Geometry: final body of the model. Coordinates: model frame, mm. Face numbers are marked on the shaded views. Round coordinates to 2 decimals unless told otherwise and drop trailing zeros. Write each loop counter-clockwise with the first axis right and the second up, starting at its lowest first coordinate (ties: lowest second). Pieces come first, ordered by that corner, then holes. Notation, with made-up numbers: (-35.5, 49.25) -> (-3.5, 49.25) arc R24 ccw to (-3.5, 87.25) -> close; hole circle Ø3 at (-29.5, -37). An arc over 180 degrees is marked (long way). Use one line per item in the form item = value. Start each with the question number.
1. Cut plane A-A, the plane z = 210. Return the cut outline in (x, y).
2. Line query: L1, parallel to X at y = 183.5, z = 282; L2, parallel to Z at x = -108, y = 96.5; L3, parallel to Y at x = -107, z = 619.5. Output: solid intervals per line, ascending.
3. Cut plane B-B, the plane x = 62. Return the cut outline in (y, z), plus the area to 3 significant figures.
4. Cut plane C-C, the plane z = 409.5. Return the cut outline in (x, y), plus the area to 3 significant figures.
5. Draft query along Y for the marked faces 1, 2 and 3. Return one class per face: pulls with the +Y half, pulls with the -Y half, needs draft (parallel to the pull), parting line crosses it, or undercut.
6. Pin query (flat end, axial travel): pin 1 Ø10 at (x, z) = (94, 382) entering from +Y; pin 2 Ø1.5 at (x, z) = (-61.5, 582) entering from +Y; pin 3 Ø4 at (x, y) = (-74.5, 30.5) entering from -Z. Return the tip coordinate at first contact, or that it passes through.
7. Cut plane D-D, the plane y = 159. Return the cut outline in (x, z), plus the area to 3 significant figures.
```python
from build123d import *

# Parameters (mm, degrees)
F0_W      = 400
F0_H      = 400
F1_DEPTH  = 400
F2_W      = 300
F2_H      = 350
F3_DEPTH  = 400.001
F4_W      = 300
F4_H      = 350
F5_DEPTH  = 400.001
F8_W      = 400
F8_H      = 330.777927181
F9_DEPTH  = 50
F10_DEPTH = 9.0852224141
F11_W     = 300
F11_H     = 150
F12_DEPTH = 176.0726081542


with BuildPart() as f1:
    # F0 (on Top) → F1 (new body)
    with BuildSketch(Plane.XY):
        Rectangle(F0_W, F0_H)
    extrude(amount=F1_DEPTH)

    # F2 (on face) → F3 (cut, through all)
    with BuildSketch(Plane.XZ.offset(200)):
        with Locations((0, 175)):
            Rectangle(F2_W, F2_H)
    extrude(amount=-F3_DEPTH, mode=Mode.SUBTRACT)

    # F4 (on face) → F5 (cut, through all)
    with BuildSketch(Plane.YZ.offset(200)):
        with Locations((0, 175)):
            Rectangle(F4_W, F4_H)
    extrude(amount=-F5_DEPTH, mode=Mode.SUBTRACT)



with BuildPart() as f9:
    # F8 (on face) → F9 (new body)
    with BuildSketch(Plane(origin=(0, 125.5652334135, -22.1405384897), x_dir=(1, 0, 0), z_dir=(0, -0.984807753, 0.1736481777))):
        with Locations((0, 594.3105737075)):
            Rectangle(F8_W, F8_H)
    extrude(amount=F9_DEPTH)


with BuildPart() as f1_1:
    add(f1.part)
    # F10 (add, through all): a face of the model
    f10_faces = [f9.part.faces().sort_by_distance(p)[0] for p in [
        (0, 175.4264955469, 404.6059930296),
    ]]

    add(f9.part)  # F10 merges F9
    extrude(f10_faces, amount=F10_DEPTH)

    # F11 (on face) → F12 (cut, through all)
    with BuildSketch(Plane(origin=(0, 76.3248457628, -13.4581296064), x_dir=(1, 0, 0), z_dir=(0, -0.984807753, 0.1736481777))):
        with Locations((0, 494.8363877028)):
            Rectangle(F11_W, F11_H)
    extrude(amount=-F12_DEPTH, mode=Mode.SUBTRACT)


solid = f1_1.part
```
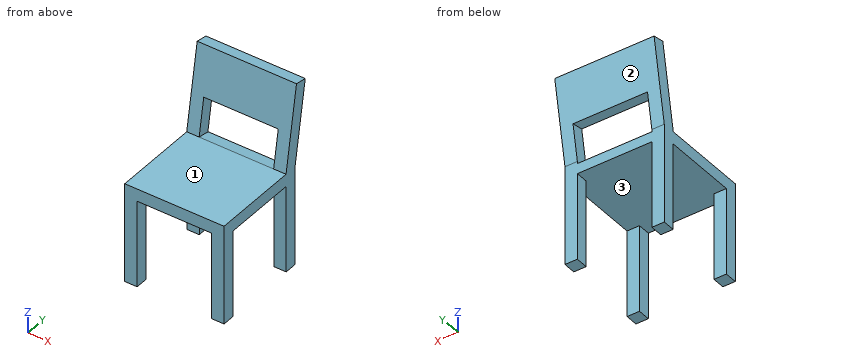
Outcome:
q1.outline = (-200, -200) -> (-150, -200) -> (-150, -150) -> (-200, -150) -> close; (-200, 150) -> (-150, 150) -> (-150, 200) -> (-200, 200) -> close; (150, -200) -> (200, -200) -> (200, -150) -> (150, -150) -> close; (150, 150) -> (200, 150) -> (200, 200) -> (150, 200) -> close
q2.L1 = -200 to -150, 150 to 200
q2.L2 = 350 to 400
q2.L3 = 187.93 to 238.7
q3.outline = (-200, 350) -> (200, 350) -> (200, 391.05) -> (149.23, 400) -> (-200, 400) -> close; (175.28, 547.72) -> (224.52, 539.04) -> (257.49, 726.02) -> (208.25, 734.7) -> close
q3.area = 29,300 mm^2
q4.outline = (-200, 150.9) -> (-150, 150.9) -> (-150, 201.68) -> (-200, 201.68) -> close; (150, 150.9) -> (200, 150.9) -> (200, 201.68) -> (150, 201.68) -> close
q4.area = 5,080 mm^2
q5.face_1 = needs draft
q5.face_2 = pulls with the +Y half
q5.face_3 = undercut
q6.pin_1 = 200
q6.pin_2 = 232.22
q6.pin_3 = 350
q7.outline = (-200, 0) -> (-150, 0) -> (-150, 350) -> (150, 350) -> (150, 0) -> (200, 0) -> (200, 455.42) -> (150, 455.42) -> (150, 398.28) -> (-150, 398.28) -> (-150, 455.42) -> (-200, 455.42) -> close
q7.area = 60,000 mm^2
